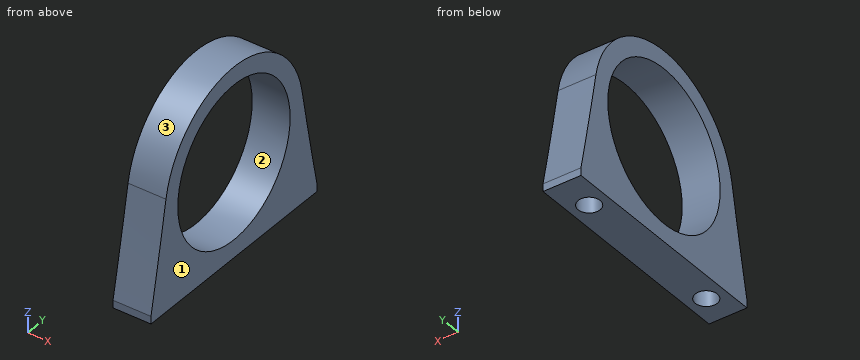
from build123d import *

# Parameters (mm, degrees)
F0_R        = 10.15
F0_W        = 30
F0_H        = 1
F1_DEPTH    = 5
F2_T1_DEPTH = 5
F3_R        = 1.45
F4_DEPTH    = 6


# Not quite as in the source:
# - a fillet or chamfer that OpenCascade refuses, or shapes differently, is made with other operations: its cross-section is extruded or revolved along the edge and cut away or added


with BuildPart() as f1:
    # F0 (on Right) → F1 (new body)
    with BuildSketch(Plane.YZ):
        with BuildLine():
            Line((15, -11.5), (12.5, 0))
            ThreePointArc((12.5, 0), (0, 12.5), (-12.5, 0))
            Line((-12.5, 0), (-15, -11.5))
            Line((-15, -11.5), (15, -11.5))
        make_face()
        Circle(F0_R, mode=Mode.SUBTRACT)
        with Locations((0, -12)):
            Rectangle(F0_W, F0_H)
    extrude(amount=F1_DEPTH)

    # F2: fillet of radius 608.1441737805 on 2 edges, made by hand

    # F2_s2 → F2_t1 (join)
    with BuildSketch(Plane.YZ):
        with BuildLine():
            ThreePointArc((-15, -11.5), (-13.6063343728, -4.6226980795), (-12.2921141837, 2.2702266177))
            ThreePointArc((-12.2921141837, 2.2702266177), (-12.4479200531, 1.1398624268), (-12.5, 0))
            Line((-12.5, 0), (-15, -11.5))
        make_face()
        with BuildLine():
            ThreePointArc((15, -11.5), (13.6063343728, -4.6226980795), (12.2921141837, 2.2702266177))
            ThreePointArc((12.2921141837, 2.2702266177), (12.4479200531, 1.1398624268), (12.5, 0))
            Line((12.5, 0), (15, -11.5))
        make_face()
    extrude(amount=F2_T1_DEPTH)

    # F3 (on face) → F4 (cut)
    with BuildSketch(Plane(origin=(0, 0, -12.5), x_dir=(1, 0, 0), z_dir=(0, 0, -1))):
        with Locations((2.4999999441, 11.0743809491)):
            Circle(F3_R)
        with Locations((2.5, -10.09248567)):
            Circle(F3_R)
    extrude(amount=-F4_DEPTH, mode=Mode.SUBTRACT)


solid = f1.part
Design review of the part built by this model. Coordinates are the model's own, in mm. Face numbers are marked on the shaded views. Coordinates: 2 decimals unless noted, no trailing zeros. Write each loop counter-clockwise with the first axis right and the second up, starting at its lowest first coordinate (ties: lowest second). Pieces come first, ordered by that corner, then holes. Notation, with made-up numbers: (-1.75, -0.5) - (17.25, -0.5) arc R29 ccw to (17.25, 26.5) - close; hole circle Ø4 at (28.5, 75). An arc over 180 degrees is marked (long way). One line per item, written item: value.
1) Add section B-B (y = -7). State the section outline as (x, z) points.
Answer sheet:
outline: (0, -12.5) - (5, -12.5) - (5, -7.35) - (0, -7.35) - close; (0, 7.35) - (5, 7.35) - (5, 10.36) - (0, 10.36) - close
2) Mouldability with a two-part tool opening along Z and no side actions: class the marked faces 1, 2 and 3 as +Z half, -Z half, draft (parallel to the pull), parting line (faces both ways), or undercut.
Answer sheet:
face 1: draft
face 2: undercut
face 3: +Z half
3) To check wall thickness, follow probe 1 along Z at (x, y) = (1.75, 0); probe 2 along Y at (x, z) = (2.5, -10.9); probe 3 along Y at (x, z) = (2.5, -9.35). State the ranges of each line that lie inside material, in increasing order.
Answer sheet:
probe 1: z = -12.5 to -10.15, 10.15 to 12.5
probe 2: y = -14.88 to -12.52, -9.62 to 8.64, 11.54 to 14.88
probe 3: y = -14.56 to -12.52, -9.62 to -3.95, 3.95 to 8.64, 11.54 to 14.56
4) Add section D-D (z = -11). State the section outline as (x, y) points, plus the area to 3 significant figures.
Answer sheet:
outline: (0, -14.9) - (5, -14.9) - (5, 14.9) - (0, 14.9) - close; hole circle Ø2.9 at (2.5, -11.07); hole circle Ø2.9 at (2.5, 10.09)
area: 136 mm2
5) Add section C-C (y = 0). State the section outline as (x, z) points, plus the area to 3 significant figures.
Answer sheet:
outline: (0, -12.5) - (5, -12.5) - (5, -10.15) - (0, -10.15) - close; (0, 10.15) - (5, 10.15) - (5, 12.5) - (0, 12.5) - close
area: 23.5 mm2
6) Insertion check: pin 1 (0.9 mm diameter, centred on x = 2.5, y = -11, fed in from -Z); pin 2 (2 mm diameter, centred on x = 3, y = -5, fed in from +Z). Each pin has a flat end and moves straight along its axis. Give the tip position at first contact, or say it passes through.
Answer sheet:
pin 1: stops at z = -6.5
pin 2: stops at z = 11.84
7) Add section A-A (x = 4.45). State the section outline as (y, z) points, plus the area to 3 significant figures.
Answer sheet:
outline: (-15, -12.5) - (15, -12.5) - (15, -11.5) arc R608.14 cw to (12.29, 2.27) arc R12.5 ccw to (-12.29, 2.27) arc R608.14 cw to (-15, -11.5) - close; hole circle Ø20.3 at (0, 0)
area: 270 mm2
